from build123d import *

# Parameters (mm, degrees)
SKETCH1_R           = 2.35
SKETCH1_R_2         = 2.5
BOSS_EXTRUDE1_DEPTH = 2.5
SKETCH2_R           = 1.5
BOSS_EXTRUDE2_DEPTH = 2.5
FILLET1_R           = 5
FILLET2_R           = 1
FILLET3_R           = 3


with BuildPart() as part:
    # Sketch1 → Boss-Extrude1 (new body)
    with BuildSketch(Plane(origin=(0, 0, 0), x_dir=(1, 0, 0), z_dir=(0, 1, 0))):
        with BuildLine():
            Line((-5.5, 0), (5.5, 0))
            Line((5.5, 0), (37.860679775, 23.511410092))
            Line((37.860679775, 23.511410092), (37.860679775, 0.360679775))
            Line((37.860679775, 0.360679775), (15, -22.5))
            ThreePointArc((15, -22.5), (0, -34.8), (-15, -22.5))
            Line((-15, -22.5), (-37.860679775, 0.360679775))
            Line((-37.860679775, 0.360679775), (-37.860679775, 23.511410092))
            Line((-37.860679775, 23.511410092), (-5.5, 0))
        make_face()
        with Locations(Location((0, -22.45, 0), (0, 0, 270))):
            Circle(SKETCH1_R, mode=Mode.SUBTRACT)
        with Locations(Location((0, -10, 0), (0, 0, 270))):
            Circle(SKETCH1_R_2, mode=Mode.SUBTRACT)
    extrude(amount=BOSS_EXTRUDE1_DEPTH)

    # Sketch2 → Boss-Extrude2 (add)
    with BuildSketch(Plane(origin=(37.860679775, 0, 0), x_dir=(0, 0, -1), z_dir=(1, 0, 0))):
        Polygon((0.360679775, 0), (25.860679775, 0), (25.860679775, 14), (6.860679775, 14), (0.360679775, 2.5), align=None)
        with Locations((6.860679775, 7.5)):
            Circle(SKETCH2_R, mode=Mode.SUBTRACT)
        with Locations((22.360679775, 11)):
            Circle(SKETCH2_R, mode=Mode.SUBTRACT)
        with Locations(Location((6.860679775, 4, 0), (0, 0, 270))):
            Circle(SKETCH2_R, mode=Mode.SUBTRACT)
    boss_extrude2 = extrude(amount=BOSS_EXTRUDE2_DEPTH)

    # Mirror1: Boss-Extrude2 across plane
    add(boss_extrude2.mirror(Plane(origin=(0, 0, 0), x_dir=(0, 0, 1), z_dir=(1, 0, 0))))

    # Fillet1
    # the kernel refuses this fillet: 5 mm, written as the material it adds along each edge
    with BuildSketch(Plane(origin=(37.860679775, 0, -23.511410092), x_dir=(-0.8090169943749437, 0, 0.5877852522924782), z_dir=(0, 1, 0))) as fillet1_piece_1:
        with BuildLine():
            CenterArc((2.542616315, -5), FILLET1_R, 90, 51.692614863)
            Line((-1.380866074, -1.900599098), (-1.459335721, -1.83861108))
            ThreePointArc((-1.459335721, -1.83861108), (-0.771334736, -0.891521024), (-0.080901699, 0.058778525))
            Line((-0.080901699, 0.058778525), (0, 0.1))
            Line((0, 0.1), (2.542616315, 0.1))
            Line((2.542616315, 0.1), (2.542616315, 0))
        make_face()
    extrude(amount=2.5)
    with BuildSketch(Plane(origin=(-37.860679775, 0, -23.511410092), x_dir=(0.8090169943749425, 0, 0.58778525229248), z_dir=(0, 1, 0))) as fillet1_piece_2:
        with BuildLine():
            CenterArc((2.542616315, 5), FILLET1_R, 218.307385137, 51.692614863)
            Line((-1.380866074, 1.900599098), (-1.459335721, 1.83861108))
            ThreePointArc((-1.459335721, 1.83861108), (-0.771334736, 0.891521024), (-0.080901699, -0.058778525))
            Line((-0.080901699, -0.058778525), (0, -0.1))
            Line((0, -0.1), (2.542616315, -0.1))
            Line((2.542616315, -0.1), (2.542616315, 0))
        make_face()
    extrude(amount=2.5)

    # Fillet2
    fillet2_edges = [part.edges().sort_by_distance(p)[0] for p in [
        (39.110679775, 2.5, -0.360679775),
        (39.110679775, 14, -25.860679775),
        (39.110679775, 14, -6.860679775),
        (-39.110679775, 2.5, -0.360679775),
        (-39.110679775, 14, -6.860679775),
        (-39.110679775, 14, -25.860679775),
    ]]
    fillet(fillet2_edges, radius=FILLET2_R)

    # Fillet3
    # the kernel refuses this fillet: 3 mm, written as the material it takes off along each edge
    with BuildSketch(Plane(origin=(-40.360679775, 0, 7.139320225), x_dir=(1, 0, 0), z_dir=(0, 0, -1)), Plane(origin=(40.360679775, 0, 7.139320225), x_dir=(0, 1, 0), z_dir=(0, 0, -1))) as fillet3_piece_1:
        with BuildLine():
            CenterArc((FILLET3_R, -FILLET3_R), FILLET3_R, 90, 90)
            Line((0, -FILLET3_R), (0, 0))
            Line((0, 0), (FILLET3_R, 0))
        make_face()
    extrude(amount=40.5, mode=Mode.SUBTRACT)


solid = part.part
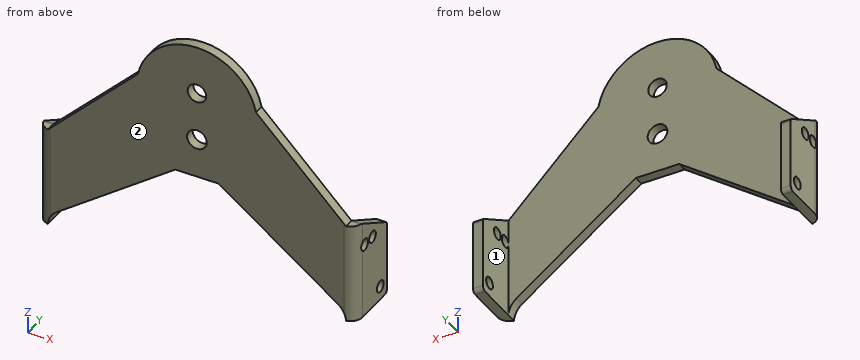
Verification items for the finished model (mm, model axes). Face numbers are marked on the shaded views. A direction names the side the tool comes from. Coordinates: 2 decimals unless noted, no trailing zeros. Write each loop counter-clockwise with the first axis right and the second up, starting at its lowest first coordinate (ties: lowest second). Pieces come first, ordered by that corner, then holes. Notation, with made-up numbers: M 22,72.25 L 58,72.25 A20 ccw 58,85.25 Z; hole C 75,54.5 d6. An arc over 180 degrees is marked long. Use CSV: the item, a comma, the result in double quotes.
Q1. Section check D-D, the plane z = 17.5. Enter the section's corners in (x, y).
Computed values:
outline,"M -20,0 L 20,0 L 20,2.5 L -20,2.5 Z"
Q2. Section check B-B, the plane y = 7.5. Enter the section's corners in (x, z), and give its area (3 significant figures).
Computed values:
outline,"M -40.36,-25.86 L -37.86,-25.86 L -37.86,-8.36 L -40.36,-8.36 Z; M -40.36,-5.36 L -37.86,-5.36 L -37.86,-3.19 L -40.36,-3.19 Z; M 37.86,-25.86 L 40.36,-25.86 L 40.36,-8.36 L 37.86,-8.36 Z; M 37.86,-5.36 L 40.36,-5.36 L 40.36,-3.19 L 37.86,-3.19 Z"
area,"98.4 mm²"
Q3. Section check C-C, the plane x = 0. Enter the section's corners in (y, z).
Computed values:
outline,"M 0,0 L 2.5,0 L 2.5,7.5 L 0,7.5 Z; M 0,12.5 L 2.5,12.5 L 2.5,20.1 L 0,20.1 Z; M 0,24.8 L 2.5,24.8 L 2.5,34.8 L 0,34.8 Z"
Q4. Set-up check for the marked faces 1 and 2: record each of +Z, -Z, +X, -X, +Y, -Y from which the full face is reachable in a straight line by a thin tool's end or side.
Computed values:
face 1,"+Z, -Z, +Y"
face 2,"+Z, -Z, +X, -X, -Y"
Q5. Go/stop test with flat-tipped pins: P1, Ø1.2, axis at x = -0.5, y = 2, coming from the -Z side; P2, Ø0.7, axis at x = 39.5, y = 1, coming from the +Z side; P3, Ø3, axis at x = -21.5, y = 3, coming from the +Z side. Record where each tip stops, or that it passes through.
Computed values:
P1,"z = 0"
P2,"z = -0.36"
P3,"z = 17.41"
Q6. Thickness scan on line 1 along X through (y, z) = (5, -3.5); line 2 along X through (y, z) = (2.25, 11.5); line 3 along Y through (x, z) = (-32, -5). Record the ranges inside material, lowest first. Write a range as [from, to].
Computed values:
line 1,"[-40.36, -37.86], [37.86, 40.36]"
line 2,"[-26, -2], [2, 26]"
line 3,"[0, 2.5]"
Q7. Section check A-A, the plane z = 10. Enter the section's corners in (x, y), and give its area (3 significant figures).
Computed values:
outline,"M -27.5,0 L -2.5,0 L -2.5,2.5 L -27.5,2.5 Z; M 2.5,0 L 27.5,0 L 27.5,2.5 L 2.5,2.5 Z"
area,"125 mm²"
